For this review, take the finished solid that the model builds, in its own axes (mm). A direction names the side the tool comes from. Coordinates: 2 decimals unless noted, no trailing zeros. Loops run counter-clockwise (first coordinate to the right, second up) from the corner with the lowest first, then second, coordinate; pieces in that order, holes last. Notation, with made-up numbers: (48.5, -14.5) - (77.5, -14.5) arc R10 cw to (77.5, -10.5) - close; hole circle Ø6 at (27.25, 5). An arc over 180 degrees is marked (long way). Answer as a JSON object with one key per item and string values. Group by question number.
Item 1: Mouldability with a two-part tool opening along Y and no side actions: class faces 1 (the flat face through (-55.937, 13, -18)), 2 (the cylindrical face through (-27.124, 0.496, -14.321)), 3 (the cylindrical face through (11.34, 28.56, -14.32)), 4 (the flat face through (-6, 58.851, -18)) as released by +Y, released by -Y, zero draft, split by the parting line, or undercut.
Item 2: Tool access review of faces 5 (the cylindrical face through (39.61, 12.82, -18.27)), 6 (the cylindrical face through (-28.596, 1.852, -19.391)): name each direction out of +Z, -Z, +X, -X, +Y, -Y from which nothing blocks a thin tool from reaching the whole face with its end or side.
Item 3: To check wall thickness, follow line 1 (Y direction, x = -5, z = -18); line 2 (Y direction, x = 10, z = -20.75); line 3 (X direction, y = -26.5, z = -15.25). State the ranges of each line that lie inside material, in increasing order.
Item 4: Clearance check with flat-ended pins moving along their axes: pin 1 (3 mm diameter, centred on x = -22, y = 2, fed in from -Z); pin 2 (4 mm diameter, centred on x = -23.83, y = 0.35, fed in from -Z). State where each tip first meets the part, or that it passes through.
Item 5: We need section A-A (z = -20.5). Give the boundary of the cut face in (x, y).
from build123d import *

# Parameters (mm, degrees)
ESBO_O1_W                = 101.9
ESBO_O1_H                = 90
RESSALTO_EXTRUS_O1_DEPTH = 10
FURO_COM_FOLGA_DE_M39_D  = 3.4
ESBO_O11_R               = 5
CORTE_EXTRUS_O1_DEPTH    = 8
FURO_COM_FOLGA_DE_M61_D  = 6.6


with BuildPart() as part:
    # Esboço1 → Ressalto-extrusão1 (new body)
    with BuildSketch(Plane.XY.offset(-23.335035958)):
        with Locations((-4.986758439, 13.850631826)):
            Rectangle(ESBO_O1_W, ESBO_O1_H)
    extrude(amount=RESSALTO_EXTRUS_O1_DEPTH)

    # Furo com folga de M39 (through all)
    with Locations(Plane(origin=(0, 0, -23.335035958), x_dir=(-1, 0, 0), z_dir=(0, 0, -1))):
        with Locations((-40.963241561, 13.850631826), (4.986758439, 53.850631826), (50.936758439, 13.850631826), (4.986758439, -26.149368174)):
            Hole(FURO_COM_FOLGA_DE_M39_D / 2)

    # Esboço11 → Corte-extrusão1 (cut)
    with BuildSketch(Plane(origin=(0, 0, -23.335035958), x_dir=(-1, 0, 0), z_dir=(0, 0, -1))):
        with Locations((-13.773241561, 26.330631826)):
            Circle(ESBO_O11_R)
        with Locations((23.826758439, 0.350631826)):
            Circle(ESBO_O11_R)
    extrude(amount=-CORTE_EXTRUS_O1_DEPTH, mode=Mode.SUBTRACT)

    # Furo com folga de M61 (through all)
    with Locations(Plane(origin=(0, 0, -15.335035958), x_dir=(-1, 0, 0), z_dir=(0, 0, -1))):
        with Locations((-13.773241561, 26.330631826), (23.826758439, 0.350631826)):
            Hole(FURO_COM_FOLGA_DE_M61_D / 2)


solid = part.part
Check sheet entries:
{
 "1": {"face 1": "zero draft", "face 2": "undercut", "face 3": "undercut", "face 4": "released by +Y"},
 "2": {"face 5": "+Z, -Z", "face 6": "-Z"},
 "3": {"line 1": "y = -31.15 to -27.85, -24.45 to 52.15, 55.55 to 58.85", "line 2": "y = -31.15 to 23.05, 29.61 to 58.85", "line 3": "x = -55.94 to -6.65, -3.32 to 45.96"},
 "4": {"pin 1": "stops at z = -15.34", "pin 2": "passes through"},
 "5": {"outline": "(-55.94, -31.15) - (45.96, -31.15) - (45.96, 58.85) - (-55.94, 58.85) - close; hole circle Ø3.4 at (-50.94, 13.85); hole circle Ø10 at (-23.83, 0.35); hole circle Ø3.4 at (-4.99, -26.15); hole circle Ø3.4 at (-4.99, 53.85); hole circle Ø10 at (13.77, 26.33); hole circle Ø3.4 at (40.96, 13.85)"}
}
